```python
from build123d import *

# Parameters (mm, degrees)
EXTRUDE_1_DEPTH     = 17
SKETCH_4_W          = 10.5
SKETCH_4_H          = 13
CUT_EXTRUDE_1_DEPTH = 1.6
SKETCH_5_W          = 0.7
SKETCH_5_H          = 0.7
CUT_EXTRUDE_2_DEPTH = 13


with BuildPart() as part:
    # 草图1 → 凸台-拉伸1 (new body)
    with BuildSketch(Plane.XY):
        Polygon((1.5, 0.044381888), (14, 0.044381888), (14, 1.344381888), (12, 2.744381888), (0, 2.744381888), (0, 1.644381888), (1.5, 1.644381888), align=None)
    extrude(amount=EXTRUDE_1_DEPTH)

    # 草图4 → 切除-拉伸1 (cut)
    with BuildSketch(Plane.XZ.offset(-0.044381888)):
        with Locations((6.75, 8.5)):
            Rectangle(SKETCH_4_W, SKETCH_4_H)
    extrude(amount=-CUT_EXTRUDE_1_DEPTH, mode=Mode.SUBTRACT)

    # 草图5 → 切除-拉伸2 (cut)
    with BuildSketch(Plane.ZY):
        with Locations((0.35, 1.294381888)):
            Rectangle(SKETCH_5_W, SKETCH_5_H)
        Polygon((0, 2.744381888), (1, 2.744381888), (1.5, 2.244381888), (2, 2.744381888), (3, 2.744381888), (3.5, 2.244381888), (4, 2.744381888), (5, 2.744381888), (5.5, 2.244381888), (6, 2.744381888), (7, 2.744381888), (7.5, 2.244381888), (8, 2.744381888), (9, 2.744381888), (9.5, 2.244381888), (10, 2.744381888), (11, 2.744381888), (11.5, 2.244381888), (12, 2.744381888), (13, 2.744381888), (13.5, 2.244381888), (14, 2.744381888), (15, 2.744381888), (15.5, 2.244381888), (16, 2.744381888), (17, 2.744381888), (17, 3.744381888), (0, 3.744381888), align=None)
        with Locations((16.65, 1.294381888)):
            Rectangle(SKETCH_5_W, SKETCH_5_H)
    extrude(amount=-CUT_EXTRUDE_2_DEPTH, mode=Mode.SUBTRACT)


solid = part.part
```
Geometry check sheet. Reference: the model listing, model coordinates, mm. A direction names the side the tool comes from. Round coordinates to 2 decimals unless told otherwise and drop trailing zeros. Order: outer loops, then holes, each group sorted by start corner. A loop starts at its lowest first (then second) coordinate and runs counter-clockwise, first axis right, second up. Notation, with made-up numbers: (-34.75, 79) - (9.25, 79) arc R25 ccw to (9.25, 108) - close; hole circle Ø10 at (35.5, 14). An arc over 180 degrees is marked (long way). Use a Markdown table: item, result. Add a question column.
1) Gauge pin test, flat ends, axial feed: P1, Ø0.8, axis at x = 4.5, y = 1.5, coming from the +Z side; P2, Ø1.3, axis at y = 0.5, z = 16, coming from the -X side; P3, Ø6.5, axis at x = 4.5, z = 6.5, coming from the -Y side; P4, Ø0.5, axis at y = 1, z = 8, coming from the -X side. Record the tip position at first contact, or that the pin passes through.
2) Set-up check for faces 5 (the flat face through (12.4, 0.044, 8.5)), 6 (the flat face through (1.5, 1, 16)): record each of +Z, -Z, +X, -X, +Y, -Y from which the full face is reachable in a straight line by a thin tool's end or side.
3) Section check C-C (y = 2). Record the cut outline in (x, z), then the cut area to 3 significant figures.
4) Section check B-B (z = 6.5). Record the cut outline in (x, y), then the cut area to 3 significant figures.
5) Mould release check, pull along Z, two halves, no side actions. Record for faces 1 (the flat face through (0, 2, 8)), 2 (the flat face through (7, 2, 17)), 3 (the flat face through (7, 1, 15)), 4 (the flat face through (7, 1, 2)): released by +Z, released by -Z, zero draft, split by the parting line, or undercut.
6) Section check A-A (y = 0.7). Record the cut outline in (x, z).
7) Thickness scan on line 1 along Z through (x, y) = (11.25, 0.25); line 2 along Z through (x, y) = (2.75, 1.2); line 3 along X through (y, z) = (0.65, 8.75). Record the ranges inside material, lowest first.
Established:
| question | item | result |
|---|---|---|
| 1 | P1 | z = 17 |
| 1 | P2 | x = 1.5 |
| 1 | P3 | y = 1.64 |
| 1 | P4 | x = 12 |
| 2 | face 5 | +Z, -Z, +X, -X, -Y |
| 2 | face 6 | +Z, -Z, -X, -Y |
| 3 | outline | (0, 0) - (13.06, 0) - (13.06, 17) - (0, 17) - close |
| 3 | area | 222 mm2 |
| 4 | outline | (0, 1.64) - (12, 1.64) - (12, 0.04) - (14, 0.04) - (14, 1.34) - (12, 2.74) - (0, 2.74) - close |
| 4 | area | 17.2 mm2 |
| 5 | face 1 | zero draft |
| 5 | face 2 | released by +Z |
| 5 | face 3 | undercut |
| 5 | face 4 | undercut |
| 6 | outline | (1.5, 0) - (14, 0) - (14, 17) - (1.5, 17) - (1.5, 15) - (12, 15) - (12, 2) - (1.5, 2) - close |
| 7 | line 1 | 0 to 2, 15 to 17 |
| 7 | line 2 | 0.7 to 2, 15 to 16.3 |
| 7 | line 3 | 12 to 14 |
